Geometry check sheet. Reference: the model listing, model coordinates, mm. Round coordinates to 2 decimals unless told otherwise and drop trailing zeros. Write each loop counter-clockwise with the first axis right and the second up, starting at its lowest first coordinate (ties: lowest second). Pieces come first, ordered by that corner, then holes. Notation, with made-up numbers: M 70.25,-17.75 L 106.25,-17.75 A20 cw 106.25,1.25 Z; hole C -2,81.5 d8. An arc over 180 degrees is marked long. Put each result on its own line as item: value. Start each with the question number.
(1) Gauge pin test, flat end, axial feed: pin 1 (1 mm diameter, centred on x = 10.5, y = 24.5, fed in from -Z). Record the tip position at first contact, or that the pin passes through.
(2) Section check A-A on x = -22. Record the cut outline in (y, z), then the cut area to 3 significant figures.
(3) Material ranges on probe 1 along Z at (x, y) = (-20, -14); probe 2 along X at (y, z) = (45, -12); probe 3 along X at (y, z) = (-17, 12), recorded low to high.
from build123d import *

# Parameters (mm, degrees)
F0_W        = 40
F0_H        = 30
F1_DEPTH    = 50
F2_R        = 5
F3_T1_DEPTH = 50
F3_T3_DEPTH = 125


# Not quite as in the source:
# - a fillet or chamfer that OpenCascade refuses, or shapes differently, is made with other operations: its cross-section is extruded or revolved along the edge and cut away or added


with BuildPart() as f1:
    # F0 (on Front) → F1 (new body, symmetric)
    with BuildSketch(Plane.XZ):
        with Locations((-4.8181314529, -0.4249101039)):
            Rectangle(F0_W, F0_H)
    extrude(amount=F1_DEPTH, both=True)

    # F2
    f2_edges = [f1.edges().sort_by_distance(p)[0] for p in [
        (-4.818131, 50, 14.57509),
        (-24.818131, 0, 14.57509),
        (-4.818131, -50, 14.57509),
        (15.181869, 0, 14.57509),
    ]]
    fillet(f2_edges, radius=F2_R)

    # F3: fillet of radius 5 on 4 edges, made by hand

    # F3_s2 → F3_t1 (cut)
    with BuildSketch(Plane.XY.offset(-27.9249101039)):
        with BuildLine():
            ThreePointArc((10.1818685471, 50), (13.717402453, 48.5355339059), (15.1818685471, 45))
            Line((15.1818685471, 45), (15.1818685471, 50))
            Line((15.1818685471, 50), (10.1818685471, 50))
        make_face()
        with BuildLine():
            ThreePointArc((15.1818685471, -45), (13.717402453, -48.5355339059), (10.1818685471, -50))
            Line((10.1818685471, -50), (15.1818685471, -50))
            Line((15.1818685471, -50), (15.1818685471, -45))
        make_face()
    extrude(amount=F3_T1_DEPTH, mode=Mode.SUBTRACT)

    # F3_s4 → F3_t3 (cut)
    with BuildSketch(Plane.XZ.offset(-62.5)):
        with BuildLine():
            ThreePointArc((15.1818685471, -10.4249101039), (13.717402453, -13.9604440098), (10.1818685471, -15.4249101039))
            Line((10.1818685471, -15.4249101039), (15.1818685471, -15.4249101039))
            Line((15.1818685471, -15.4249101039), (15.1818685471, -10.4249101039))
        make_face()
    extrude(amount=F3_T3_DEPTH, mode=Mode.SUBTRACT)


solid = f1.part
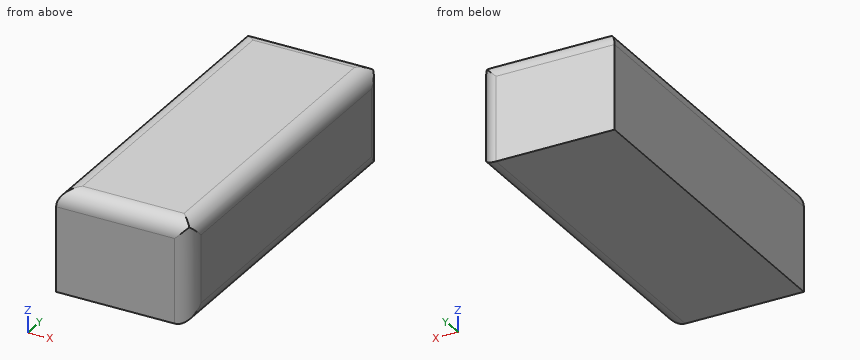
Answers follow:
1. pin 1: stops at z = -15.42
2. outline: M -50,-15.42 L 50,-15.42 L 50,9.58 A5 ccw 47.18,14.07 L -47.18,14.07 A5 ccw -50,9.58 Z
2. area: 2,940 mm^2
3. probe 1: z = -15.42 to 14.57
3. probe 2: x = -24.82 to 14.93
3. probe 3: x = -24.19 to 14.55
